Part model, mm, in its own coordinate system. A direction names the side the tool comes from. Round coordinates to 2 decimals unless told otherwise and drop trailing zeros. Loops run counter-clockwise (first coordinate to the right, second up) from the corner with the lowest first, then second, coordinate; pieces in that order, holes last.
from build123d import *

# Parameters (mm, degrees)
SKETCH_R     = 1.55
SKETCH_W     = 14
SKETCH_H     = 12
PAD_DEPTH    = 3
FILLET_R     = 0.75
POCKET_DEPTH = 5
FILLET001_R  = 0.5
CHAMFER_SIZE = 1
PAD001_DEPTH = 3
FILLET002_R  = 2
SKETCH004_W  = 0.400118
SKETCH004_H  = 2.725121
PAD002_DEPTH = 0.2


with BuildPart() as part:
    # Sketch → Pad (new body)
    with BuildSketch(Plane.XY):
        Polygon((-9.75, -9.75), (9.75, -9.75), (9.75, 9.75), (-9.75, 9.75), (-21, 9.75), (-21, -0.75), (-21.75, -0.75), (-29.75, -2.75), (-29.75, -3.75), (-3, -3.75), (-3, -5.75), (-29.75, -5.75), (-29.75, -6.75), (-21.75, -9.75), align=None)
        with Locations((0, 6)):
            Circle(SKETCH_R, mode=Mode.SUBTRACT)
        with Locations((0, -6)):
            Circle(SKETCH_R, mode=Mode.SUBTRACT)
        with Locations((-10, 3)):
            Rectangle(SKETCH_W, SKETCH_H, mode=Mode.SUBTRACT)
    extrude(amount=PAD_DEPTH)

    # Fillet
    fillet_edges = [part.edges().sort_by_distance(p)[0] for p in [
        (-3, -3, 1.5),
        (-3, 9, 1.5),
        (-17, 9, 1.5),
        (-17, -3, 1.5),
        (-3, -3.75, 1.5),
        (-3, -5.75, 1.5),
    ]]
    fillet(fillet_edges, radius=FILLET_R)

    # Sketch002 (on Face26 of Fillet) → Pocket (cut)
    with BuildSketch(Plane.XY.offset(3)):
        with BuildLine():
            ThreePointArc((-18.4, -9.353833), (-19, -8.753833), (-19.6, -9.353833))
            Line((-19.6, -9.353833), (-19.6, -11.103725))
            ThreePointArc((-19.6, -11.103725), (-19, -11.703725), (-18.4, -11.103725))
            Line((-18.4, -9.353833), (-18.4, -11.103725))
        make_face()
        with BuildLine():
            ThreePointArc((-18.4, 12.382466), (-19, 12.982466), (-19.6, 12.382466))
            Line((-19.6, 12.382466), (-19.6, 9.326973))
            ThreePointArc((-19.6, 9.326973), (-19, 8.726973), (-18.4, 9.326973))
            Line((-18.4, 12.382466), (-18.4, 9.326973))
        make_face()
    extrude(amount=-POCKET_DEPTH, mode=Mode.SUBTRACT)

    # Fillet001
    fillet001_edges = [part.edges().sort_by_distance(p)[0] for p in [
        (-21, 9.75, 1.5),
        (-21, -0.75, 1.5),
        (9.75, -9.75, 1.5),
        (9.75, 9.75, 1.5),
        (-19.6, 9.75, 1.5),
        (-18.4, 9.75, 1.5),
        (-19.6, -9.75, 1.5),
        (-18.4, -9.75, 1.5),
        (-29.75, -6.75, 1.5),
        (-29.75, -2.75, 1.5),
    ]]
    fillet(fillet001_edges, radius=FILLET001_R)

    # Chamfer
    chamfer_edges = [part.edges().sort_by_distance(p)[0] for p in [
        (-1.55, 6, 3),
        (-1.55, -6, 3),
    ]]
    chamfer(chamfer_edges, length=CHAMFER_SIZE)

    # Sketch003 (on Face4 of Chamfer) → Pad001 (join)
    with BuildSketch(Plane.XY.offset(3)):
        Polygon((-14.75, 9), (-13.017949, 8), (-6.982051, 8), (-5.25, 9), align=None)
        Polygon((-14.75, -3), (-13.017949, -2), (-6.982051, -2), (-5.25, -3), align=None)
    extrude(amount=-PAD001_DEPTH)

    # Fillet002
    fillet002_edges = [part.edges().sort_by_distance(p)[0] for p in [
        (-5.25, -3, 1.5),
        (-14.75, -3, 1.5),
        (-13.017949, -2, 1.5),
        (-6.982051, -2, 1.5),
        (-5.25, 9, 1.5),
        (-6.982051, 8, 1.5),
        (-13.017949, 8, 1.5),
        (-14.75, 9, 1.5),
    ]]
    fillet(fillet002_edges, radius=FILLET002_R)

    # Sketch004 (on Face1 of Fillet002) → Pad002 (join)
    with BuildSketch(Plane(origin=(0, 0, 0), x_dir=(1, 0, 0), z_dir=(0, 0, -1))):
        with Locations((-25.583762, 4.610938)):
            Rectangle(SKETCH004_W, SKETCH004_H)
    extrude(amount=-PAD002_DEPTH)


solid = part.part
1) Slice it at C-C, the plane x = -23.5. Give the cut face in (y, z).
Values:
outline: (-9.09, 0) - (-5.75, 0) - (-5.75, 3) - (-9.09, 3) - close; (-3.75, 0) - (-1.19, 0) - (-1.19, 3) - (-3.75, 3) - close
2) Slice it at B-B, the plane y = 6. Give the cut face in (x, z), then the cut area to 4 significant figures.
Values:
outline: (-21, 0) - (-17, 0) - (-17, 3) - (-21, 3) - close; (-3, 0) - (-1.55, 0) - (-1.55, 2) - (-2.55, 3) - (-3, 3) - close; (1.55, 0) - (9.75, 0) - (9.75, 3) - (2.55, 3) - (1.55, 2) - close
area: 39.95 mm2
3) Slice it at A-A, the plane x = -11. Give the cut face in (y, z).
Values:
outline: (-9.75, 0) - (-5.75, 0) - (-5.75, 3) - (-9.75, 3) - close; (-3.75, 0) - (-2, 0) - (-2, 3) - (-3.75, 3) - close; (8, 0) - (9.75, 0) - (9.75, 3) - (8, 3) - close
4) Tool access for faces 4 (the face through (-25.64, -8.29, 1.48)), 5 (the face through (-5.225, 8.934, 1.479)): list every direction of +Z, -Z, +X, -X, +Y, -Y with a clear straight run to the whole face (end or side of a thin tool).
Values:
face 4: +Z, -Z, -X, -Y
face 5: +Z, -Z
5) Drop a flat-ended pin along its axis: pin 1 Ø3 at (x, y) = (0, 6) entering from -Z. Give the stop position or say it passes through.
Values:
pin 1: passes through
6) Slice it at D-D, the plane y = -1.5. Give the cut face in (x, z), then the cut area to 3 significant figures.
Values:
outline: (-24.75, 0) - (-17, 0) - (-17, 3) - (-24.75, 3) - close; (-3, 0) - (9.75, 0) - (9.75, 3) - (-3, 3) - close
area: 61.5 mm2
7) Wall check: line 1 along Y through (x, z) = (-9, 2.2); line 2 along Y through (x, z) = (0, 1); line 3 along Y through (x, z) = (-18, 0.9). Give the ranges that are in metal, low to high.
Values:
line 1: y = -9.75 to -5.75, -3.75 to -2, 8 to 9.75
line 2: y = -9.75 to -7.55, -4.45 to 4.45, 7.55 to 9.75
line 3: y = -9.74 to -5.75, -3.75 to 9.74
8) Mould opens along X. For faces 1 (the face through (-25.51, -1.69, 1.48)), 2 (the face through (-1, -2, 3)), 3 (the face through (-14.775, -2.934, 1.479)) say: released by +X, released by -X, zero draft, split by the parting line, or undercut.
Values:
face 1: released by -X
face 2: zero draft
face 3: undercut
